Part model, mm, in its own coordinate system. Face numbers are marked on the shaded views. A direction names the side the tool comes from. Round coordinates to 2 decimals unless told otherwise and drop trailing zeros. Write each loop counter-clockwise with the first axis right and the second up, starting at its lowest first coordinate (ties: lowest second). Pieces come first, ordered by that corner, then holes. Notation, with made-up numbers: (29.25, -24) -> (36.25, -24) arc R28 ccw to (36.25, 14) -> close; hole circle Ø3 at (3.5, 14). An arc over 180 degrees is marked (long way). Return JSON: item names as keys, results as strings. Group by question number.
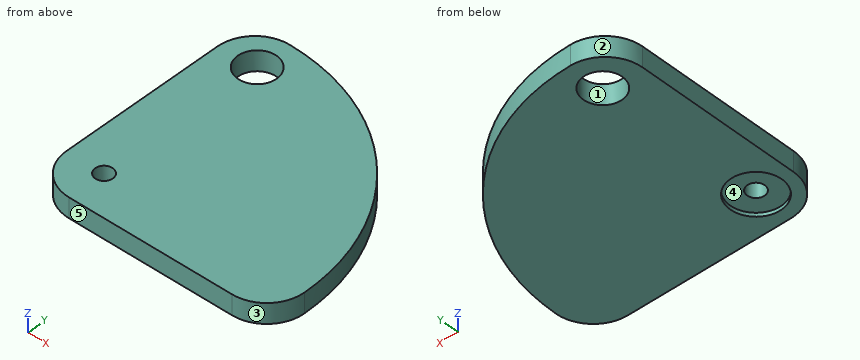
Autodesk Fusion 360 part; units mm, degrees
sketch "Smartie Arm" plane through (0, 0, 0) normal (0, 0, 1) x (1, 0, 0)
  line L0 (0, 0) -> (95, 0)
  line L1 (95, 0) -> (95, 95)
  line L2 (95, 95) -> (0, 95)
  line L3 (0, 95) -> (0, 0)
  dimension "d6" = 95
  dimension "d15" = 95
extrude "Extrude1" add sketch "Smartie Arm" along normal blind 8
sketch "Smartie Hole" plane through (0, 0, 8) normal (0, 0, 1) x (-1, 0, 0)
  line L0 (0, -95) -> (0, 0)
  line L1 (0, 0) -> (-95, 0)
  line L2 (-95, 0) -> (-95, -95)
  line L3 (-95, -95) -> (0, -95)
  circle A0 centre (-15, -81) radius 7.75
  dimension "d5" = 15.5
  dimension "d8" = 15
  dimension "d9" = 80
  dimension "d14" = 14
extrude "Extrude2" cut sketch "Smartie Hole" against normal blind 8 contours A0
fillet "Fillet1" radius 15 2 edges at (95, 95, 4) (0, 95, 4)
fillet "Fillet2" radius 15 2 edges at (0, 0, 4) (95, 0, 4)
sketch "Smartie Arm Arc" plane through (0, 0, 8) normal (0, 0, 1) x (-1, 0, 0)
  arc A0 (-80, 0) -> (-95, -15) centre (-80, -15) ccw
  line L0 (-95, -15) -> (-95, -80)
  arc A1 (-95, -80) -> (-80, -95) centre (-80, -80) ccw
  line L1 (-80, -95) -> (-15, -95)
  arc A2 (-15, -95) -> (0, -80) centre (-15, -80) ccw
  line L2 (0, -80) -> (0, -15)
  arc A3 (0, -15) -> (-15, 0) centre (-15, -15) ccw
  line L3 (-15, 0) -> (-80, 0)
  circle A4 centre (-15, -81) radius 7.75
  circle A5 centre (-15, -15) radius 80
  dimension "d16" = 15
  dimension "d17" = 15
  dimension "d18" = 160
extrude "Extrude3" cut sketch "Smartie Arm Arc" against normal blind 8 contours L0 A1 L1 A5
sketch "Servo Horn Hole" plane through (0, 0, 0) normal (0, 0, -1) x (1, 0, 0)
  arc A0 (15, -95) -> (95, -15) centre (15, -15) ccw
  arc A1 (95, -15) -> (80, 0) centre (80, -15) ccw
  line L0 (80, 0) -> (15, 0)
  arc A2 (15, 0) -> (0, -15) centre (15, -15) ccw
  line L1 (0, -15) -> (0, -80)
  arc A3 (0, -80) -> (15, -95) centre (15, -80) ccw
  circle A4 centre (15, -81) radius 7.75
  circle A5 centre (15, -15) radius 10.25
  circle A6 centre (15, -15) radius 3.5
  dimension "d21" = 20.5
  dimension "d24" = 7
extrude "Extrude4" cut sketch "Servo Horn Hole" against normal blind 1.5 contours A5 | A6
extrude "Extrude5" cut sketch "Servo Horn Hole" against normal blind 8 contours A6
equation "d14 = 16 mm - 2 mm"
Item 1: Wall check: L1, parallel to Y at x = 15, z = 2.75; L2, parallel to Y at x = 15, z = 0.55; L3, parallel to X at y = 15, z = 1.1. Give the ranges that are in metal, low to high.
Item 2: Two-plate mould, pull along X, no slides. Class the marked faces 1, 2 and 3: released by +X, released by -X, zero draft, split by the parting line, or undercut.
Item 3: Which spindle directions (+Z, -Z, +X, -X, +Y, -Y) get a long thin tool onto all of the face, cutting with end or side? Do the marked faces 4 and 5. Say none if no direction does.
Item 4: Flat gauge pins, fed straight in: P1, Ø9.5, axis at x = 15, y = 81, coming from the +Z side; P2, Ø1.5, axis at y = 70, z = 3, coming from the +X side. Where does each tip first touch, or does it go through?
Item 5: Cut at A-A (z = 5.25). Write the cut outline in (x, y).
Item 6: Cut at D-D (x = 67.5). Write the cut outline in (y, z).
Item 7: Cut at B-B (y = 84). Write the cut outline in (x, z).
Item 8: Cut at C-C (y = 46). Write the cut outline in (x, z), then the cut area to 3 significant figures.
Checks:
{
 "1": {"L1": "y = 0 to 11.5, 18.5 to 73.25, 88.75 to 95", "L2": "y = 0 to 4.75, 25.25 to 73.25, 88.75 to 95", "L3": "x = 0 to 4.75, 25.25 to 95"},
 "2": {"face 1": "undercut", "face 2": "released by -X", "face 3": "released by +X"},
 "3": {"face 4": "-Z", "face 5": "+Z, -Z, +X, -X, -Y"},
 "4": {"P1": "passes through", "P2": "stops at x = 73.8"},
 "5": {"outline": "(0, 15) arc R15 ccw to (15, 0) -> (80, 0) arc R15 ccw to (95, 15) arc R80 ccw to (15, 95) arc R15 ccw to (0, 80) -> close; hole circle Ø15.5 at (15, 81); hole circle Ø7 at (15, 15)"},
 "6": {"outline": "(0, 0) -> (75.36, 0) -> (75.36, 8) -> (0, 8) -> close"},
 "7": {"outline": "(0.54, 0) -> (7.85, 0) -> (7.85, 8) -> (0.54, 8) -> close; (22.15, 0) -> (55.48, 0) -> (55.48, 8) -> (22.15, 8) -> close"},
 "8": {"outline": "(0, 0) -> (88.75, 0) -> (88.75, 8) -> (0, 8) -> close", "area": "710 mm2"}
}
